Geometry check sheet. Reference: the model listing, model coordinates, mm. A direction names the side the tool comes from. Coordinates: 2 decimals unless noted, no trailing zeros. Write each loop counter-clockwise with the first axis right and the second up, starting at its lowest first coordinate (ties: lowest second). Pieces come first, ordered by that corner, then holes. Notation, with made-up numbers: (15.25, -34.75) -> (41.25, -34.75) arc R23 ccw to (41.25, -0.75) -> close; hole circle Ø11 at (58.5, 42.5). An arc over 180 degrees is marked (long way). Answer in a Markdown table with one row per item. Add a question column.
1. Depth check by flat-ended pin: P1, Ø6, axis at x = 5, y = -43.5, coming from the -Z side; P2, Ø1.2, axis at y = -6.5, z = 0.5, coming from the +X side; P3, Ø16, axis at y = -28, z = -20.5, coming from the -X side; P4, Ø0.5, axis at x = 7.5, z = -7, coming from the +Y side. Enter the tip coordinate at first touch or a pass-through.
2. Cross-section at B-B on y = 0. Record the cut outline in (x, z).
3. Cross-section at D-D on y = -50.5. Record the cut outline in (x, z), and give its area (3 significant figures).
4. Set-up check for faces 4 (the cylindrical face through (5.58, -28.05, -30.13)), 5 (the cylindrical face through (7, 0, 4)), 6 (the flat face through (7, 7, 2)), 7 (the cylindrical face through (7, -4, 0)), 8 (the flat face through (7, -7, 2)): record each of +Z, -Z, +X, -X, +Y, -Y from which the full face is reachable in a straight line by a thin tool's end or side.
5. Mould release check, pull along Y, two halves, no side actions. Record for faces 1 (the flat face through (2, -7, 1)), 2 (the flat face through (-3, 0, 0)), 3 (the cylindrical face through (7, 4, 0)): pulls with the +Y half, pulls with the -Y half, needs draft (parallel to the pull), parting line crosses it, or undercut.
6. Scan lines: L1, parallel to Y at x = -0.3, z = 0; L2, parallel to Y at x = 1.5, z = -1; L3, parallel to Z at x = -0.05, y = -6. Record each from-to range of solid material in increasing order. Write a range as from..to.
7. Cross-section at C-C on y = -13. Record the cut outline in (x, z), and give its area (3 significant figures).
8. Cross-section at A-A on z = -23. Record the cut outline in (x, y).
```python
from build123d import *

# Parameters (mm, degrees)
HUB_SKETCH_R    = 8
HUB_SKETCH_R_2  = 1.15
HUB_DEPTH       = 11
HUB_DEPTH_BACK  = 3
LEG_DEPTH       = 11
CLEARANCE_DEPTH = 9
FILLET_2_R      = 0.75


with BuildPart() as part:
    # Hub-Sketch → Hub (new body, two sides)
    with BuildSketch(Plane(origin=(0, 0, 0), x_dir=(0, 0, -1), z_dir=(1, 0, 0))) as hub_sk:
        Circle(HUB_SKETCH_R)
        with Locations((0, 6)):
            Circle(HUB_SKETCH_R_2, mode=Mode.SUBTRACT)
        with Locations((-6, 0)):
            Circle(HUB_SKETCH_R_2, mode=Mode.SUBTRACT)
        with Locations((0, -6)):
            Circle(HUB_SKETCH_R_2, mode=Mode.SUBTRACT)
        with Locations((6, 0)):
            Circle(HUB_SKETCH_R_2, mode=Mode.SUBTRACT)
    extrude(amount=HUB_DEPTH)
    extrude(hub_sk.sketch, amount=-HUB_DEPTH_BACK)

    # Leg-Sketch → Leg (add)
    with BuildSketch(Plane(origin=(11, 0, 0), x_dir=(0, 0, -1), z_dir=(1, 0, 0))):
        with BuildLine():
            Line((0, -56), (0, -54.4))
            ThreePointArc((0, -54.4), (30.279762218, -26.701110883), (5.380854951, 5.92))
            ThreePointArc((5.380854951, 5.92), (2.88444102, 7.461903242), (0, 8))
            ThreePointArc((0, 8), (32, -24), (0, -56))
        make_face()
    extrude(amount=-LEG_DEPTH)

    # Clearance-Sketch → Clearance (cut)
    with BuildSketch(Plane(origin=(11, 0, 0), x_dir=(0, 0, -1), z_dir=(1, 0, 0))):
        with BuildLine():
            Line((-2, 8), (2, 8))
            Line((2, 8), (2, 6))
            ThreePointArc((2, 6), (0, 4), (-2, 6))
            Line((-2, 6), (-2, 8))
        make_face()
        with BuildLine():
            Line((8, 2), (8, -2))
            Line((8, -2), (6, -2))
            ThreePointArc((6, -2), (4, 0), (6, 2))
            Line((6, 2), (8, 2))
        make_face()
        with BuildLine():
            Line((2, -8), (-2, -8))
            Line((-2, -8), (-2, -6))
            ThreePointArc((-2, -6), (0, -4), (2, -6))
            Line((2, -6), (2, -8))
        make_face()
        with BuildLine():
            Line((-8, -2), (-8, 2))
            Line((-8, 2), (-6, 2))
            ThreePointArc((-6, 2), (-4, 0), (-6, -2))
            Line((-6, -2), (-8, -2))
        make_face()
    extrude(amount=-CLEARANCE_DEPTH, mode=Mode.SUBTRACT)

    # Fillet 2
    fillet_2_edges = [part.edges().sort_by_distance(p)[0] for p in [
        (5.5, 5.92, -5.380854951),
        (5.5, -56, 0),
        (5.5, -54.4, 0),
    ]]
    fillet(fillet_2_edges, radius=FILLET_2_R)


solid = part.part
```
Results found:
| question | item | result |
|---|---|---|
| 1 | P1 | stops at z = -27.42 |
| 1 | P2 | stops at x = 2 |
| 1 | P3 | passes through |
| 1 | P4 | stops at y = 7.28 |
| 2 | outline | (-3, -8) -> (2, -8) -> (2, -7.15) -> (-3, -7.15) -> close; (-3, -4.85) -> (2, -4.85) -> (2, -4) -> (11, -4) -> (11, 4) -> (2, 4) -> (2, 4.85) -> (-3, 4.85) -> close; (-3, 7.15) -> (2, 7.15) -> (2, 8) -> (-3, 8) -> close; (0, -21.17) -> (11, -21.17) -> (11, -18.66) -> (0, -18.66) -> close |
| 3 | outline | (0, -17.94) -> (11, -17.94) -> (11, -14.9) -> (0, -14.9) -> close |
| 3 | area | 33.4 mm^2 |
| 4 | face 4 | +X, -X |
| 4 | face 5 | +Z, +X |
| 4 | face 6 | +X, +Y |
| 4 | face 7 | +X |
| 4 | face 8 | +X, -Y |
| 5 | face 1 | undercut |
| 5 | face 2 | needs draft |
| 5 | face 3 | pulls with the +Y half |
| 6 | L1 | y = -8..-7.15, -4.85..4.85, 7.15..8 |
| 6 | L2 | y = -55.98..-54.38, -7.94..-6.57, -5.43..5.43, 6.57..7.98 |
| 6 | L3 | z = -5.29..-1.15, 1.15..5.29 |
| 7 | outline | (0, -30.05) -> (11, -30.05) -> (11, -28.34) -> (0, -28.34) -> close |
| 7 | area | 18.8 mm^2 |
| 8 | outline | (0, -46.25) -> (11, -46.25) -> (11, -43.88) -> (0, -43.88) -> close; (0, -4.12) -> (11, -4.12) -> (11, -1.75) -> (0, -1.75) -> close |
